```python
from build123d import *

# Parameters (mm, degrees)
F1_DEPTH = 10
F2_R     = 20
F3_DEPTH = 5
F4_R     = 10
F5_DEPTH = 25


with BuildPart() as f1:
    # F0 (on Top) → F1 (new body)
    with BuildSketch(Plane.XY):
        Polygon((25, -10.355339), (25, 10.355339), (10.355339, 25), (-10.355339, 25), (-25, 10.355339), (-25, -10.355339), (-10.355339, -25), (10.355339, -25), align=None)
    extrude(amount=F1_DEPTH)

    # F2 (on face) → F3 (cut)
    with BuildSketch(Plane.XY.offset(10)):
        Circle(F2_R)
    extrude(amount=-F3_DEPTH, mode=Mode.SUBTRACT)

    # F4 (on face) → F5 (cut)
    with BuildSketch(Plane.XY.offset(10)):
        Circle(F4_R)
    extrude(amount=-F5_DEPTH, mode=Mode.SUBTRACT)


solid = f1.part
```
Part model, mm, in its own coordinate system. A direction names the side the tool comes from. Round coordinates to 2 decimals unless told otherwise and drop trailing zeros. Loops run counter-clockwise (first coordinate to the right, second up) from the corner with the lowest first, then second, coordinate; pieces in that order, holes last.
1. Drill centre lines: line 1 along Y through (x, z) = (0, 7.5); line 2 along Y through (x, z) = (0, 3.5); line 3 along Z through (x, y) = (7.5, 17.5). Where is each one in solid material? Low to high.
Solutions:
line 1: y = -25 to -20, 20 to 25
line 2: y = -25 to -10, 10 to 25
line 3: z = 0 to 5
2. Slice it at D-D (x = 15.5). Give the cut face in (y, z).
Solutions:
outline: (-19.86, 0) - (19.86, 0) - (19.86, 10) - (12.64, 10) - (12.64, 5) - (-12.64, 5) - (-12.64, 10) - (-19.86, 10) - close
3. Slice it at A-A (y = 0). Give the cut face in (x, z), and give its area (3 significant figures).
Solutions:
outline: (-25, 0) - (-10, 0) - (-10, 5) - (-20, 5) - (-20, 10) - (-25, 10) - close; (10, 0) - (25, 0) - (25, 10) - (20, 10) - (20, 5) - (10, 5) - close
area: 200 mm2
4. 3-axis set-ups, long thin cutter, end or side, ignore diameter. For faces 1 (the face through (17.575, -17.78, 4.93)), 2 (the face through (-5, 9, 5)): which of +Z, -Z, +X, -X, +Y, -Y reach the whole face in a straight line?
Solutions:
face 1: +Z, -Z, +X, -Y
face 2: +Z
5. Two-plate mould, pull along Y, no slides. Class faces 3 (the face through (0, -25, 5)), 4 (the face through (0, 25, 5)), 5 (the face through (-2.17, -9.76, 2.54)): pulls with the +Y half, pulls with the -Y half, needs draft (parallel to the pull), parting line crosses it, or undercut.
Solutions:
face 3: pulls with the -Y half
face 4: pulls with the +Y half
face 5: undercut
6. Slice it at C-C (z = 6.25). Give the cut face in (x, y), and give its area (3 significant figures).
Solutions:
outline: (-25, -10.36) - (-10.36, -25) - (10.36, -25) - (25, -10.36) - (25, 10.36) - (10.36, 25) - (-10.36, 25) - (-25, 10.36) - close; hole circle Ø40 at (0, 0)
area: 814 mm2
7. Flat gauge pins, fed straight in: pin 1 (8 mm diameter, centred on x = -7.5, y = 17.5, fed in from +Z); pin 2 (6 mm diameter, centred on x = 8.5, y = -2, fed in from +Z); pin 3 (1.5 mm diameter, centred on x = -17, z = 9, fed in from +Y). Where does each tip first touch, or does it go through?
Solutions:
pin 1: stops at z = 10
pin 2: stops at z = 5
pin 3: stops at y = 19.11
